from build123d import *

# Parameters (mm, degrees)
BOSS_EXTRUDE1_DEPTH             = 14
FILLET1_RADIUS                  = 7
FILLET1_LENGTH                  = 1.6
F_8_0MM_DOWEL_HOLE2_D           = 8
F_8_0MM_DOWEL_HOLE2_DEPTH       = 30
F_8_0MM_DOWEL_HOLE2_CSINK_D     = 8.05
F_8_0MM_DOWEL_HOLE2_CSINK_ANGLE = 90
F_8_0MM_DOWEL_HOLE2_TIP         = 2.403442476
F_3_0MM_DOWEL_HOLE1_D           = 3
F_3_0MM_DOWEL_HOLE1_DEPTH       = 30
F_3_0MM_DOWEL_HOLE1_CSINK_D     = 3.05
F_3_0MM_DOWEL_HOLE1_CSINK_ANGLE = 90
F_3_0MM_DOWEL_HOLE1_TIP         = 0.901290929
FILLET2_R                       = 5
FILLET3_R                       = 2


with BuildPart() as part:
    # Sketch1 → Boss-Extrude1 (new body)
    with BuildSketch(Plane.XY):
        Polygon((0, 0), (21.6, 0), (21.6, 30), (20, 30), (20, 1.6), (0, 1.6), align=None)
    extrude(amount=BOSS_EXTRUDE1_DEPTH)

    # Fillet1: full round fillet: the end face becomes a half cylinder, R = half its width
    fillet1_face = Plane((0, 0.8, 7), x_dir=(0, 1, 0), z_dir=(-1, 0, 0))  # on the end face: x along it, z out of the body
    fillet1_slab = fillet1_face.offset(-FILLET1_RADIUS / 2) * Box(FILLET1_LENGTH, 2 * FILLET1_RADIUS, FILLET1_RADIUS, mode=Mode.PRIVATE)  # the body's end, R deep
    fillet1_round = Plane((7, 0.8, 7), x_dir=(-1, 0, 0), z_dir=(0, 1, 0)) * Cylinder(FILLET1_RADIUS, FILLET1_LENGTH, mode=Mode.PRIVATE)  # its axis R under the face
    add(fillet1_slab - fillet1_round, mode=Mode.SUBTRACT)

    # Ø8.0mm Dowel Hole2
    with Locations(Plane(origin=(0, 1.6, 0), x_dir=(1, 0, 0), z_dir=(0, 1, 0))):
        with Locations((7, -7)):
            CounterSinkHole(F_8_0MM_DOWEL_HOLE2_D / 2, F_8_0MM_DOWEL_HOLE2_CSINK_D / 2, depth=F_8_0MM_DOWEL_HOLE2_DEPTH, counter_sink_angle=F_8_0MM_DOWEL_HOLE2_CSINK_ANGLE)
            with Locations((0, 0, -(F_8_0MM_DOWEL_HOLE2_DEPTH + F_8_0MM_DOWEL_HOLE2_TIP / 2))):  # 118° drill point
                Cone(0, F_8_0MM_DOWEL_HOLE2_D / 2, F_8_0MM_DOWEL_HOLE2_TIP, mode=Mode.SUBTRACT)

    # Ø3.0mm Dowel Hole1
    with Locations(Plane.ZY.offset(-20)):
        with Locations((7, 24), (7, 17)):
            CounterSinkHole(F_3_0MM_DOWEL_HOLE1_D / 2, F_3_0MM_DOWEL_HOLE1_CSINK_D / 2, depth=F_3_0MM_DOWEL_HOLE1_DEPTH, counter_sink_angle=F_3_0MM_DOWEL_HOLE1_CSINK_ANGLE)
            with Locations((0, 0, -(F_3_0MM_DOWEL_HOLE1_DEPTH + F_3_0MM_DOWEL_HOLE1_TIP / 2))):  # 118° drill point
                Cone(0, F_3_0MM_DOWEL_HOLE1_D / 2, F_3_0MM_DOWEL_HOLE1_TIP, mode=Mode.SUBTRACT)

    # Fillet2
    fillet2_edges = [part.edges().sort_by_distance(p)[0] for p in [
        (20.8, 30, 14),
        (20.8, 30, 0),
    ]]
    fillet(fillet2_edges, radius=FILLET2_R)

    # Fillet3
    fillet3_edges = [part.edges().sort_by_distance(p)[0] for p in [
        (20, 1.6, 7),
        (21.6, 0, 7),
    ]]
    fillet(fillet3_edges, radius=FILLET3_R)


solid = part.part
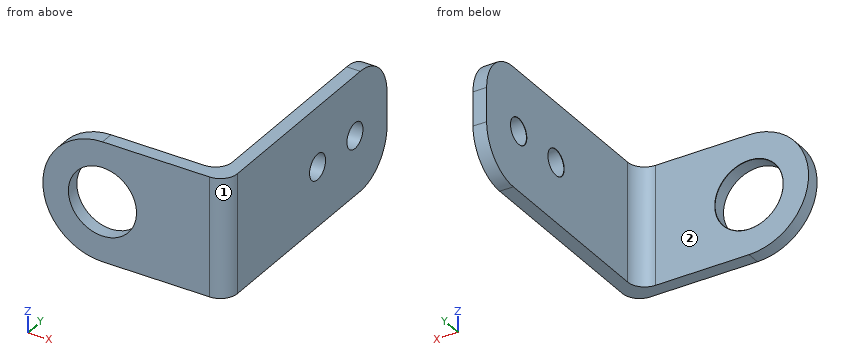
Verification items for the finished model (mm, model axes). Face numbers are marked on the shaded views. A direction names the side the tool comes from. Give positions to 0.01 mm unless a question says otherwise; leave off trailing zeros. Write each loop counter-clockwise with the first axis right and the second up, starting at its lowest first coordinate (ties: lowest second). Pieces come first, ordered by that corner, then holes.
(1) Cross-section at C-C (z = 7.75). State how many separate pieces and enclosed holes the cut face has, plus the area to 3 significant figures.
(2) Cross-section at A-A (y = 24). Enter the section's corners in (x, z) (3 decimals), plus the area to 3 significant figures.
(3) Material ranges on line 1 (Z direction, x = 20.35, y = 24); line 2 (Z direction, x = 7, y = 0.9); line 3 (Y direction, x = 13, z = 7.5), recorded low to high.
(4) Cross-section at B-B (y = 12.75). Enter the section's corners in (x, z), plus the area to 3 significant figures.
(5) Cross-section at D-D (x = 2). Enter the section's corners in (y, z).
(6) Gauge pin test, flat ends, axial feed: pin 1 (4 mm diameter, centred on y = 6, z = 11, fed in from -X); pin 2 (5 mm diameter, centred on x = 4, z = 1.5, fed in from +Y). Record the tip position at first contact, or that the pin passes through.
(7) Access from +Z, -Z, +X, -X, +Y, -Y to the whole of each face (thin tool, end or side, straight path). Record for the marked faces 1 and 2.
Worked out:
1. separate pieces: 4
1. enclosed holes: 0
1. area: 59.0 mm2
2. outline: (20, 0) - (21.6, 0) - (21.6, 5.5) - (20.025, 5.5) - (20, 5.475) - close; (20, 8.525) - (20.025, 8.5) - (21.6, 8.5) - (21.6, 14) - (20, 14) - close
2. area: 17.6 mm2
3. line 1: z = 0 to 5.5, 8.5 to 14
3. line 2: z = 0 to 3, 11 to 14
3. line 3: y = 0 to 1.6
4. outline: (20, 0) - (21.6, 0) - (21.6, 14) - (20, 14) - close
4. area: 22.4 mm2
5. outline: (0, 2.1) - (1.6, 2.1) - (1.6, 11.9) - (0, 11.9) - close
6. pin 1: stops at x = 20
6. pin 2: stops at y = 1.6
7. face 1: +Z, -Z, +X, -Y
7. face 2: +Z, -Z, -X, +Y
